from build123d import *

# Parameters (mm, degrees)
EXTRUDE086_DEPTH = 0.8
EXTRUDE087_DEPTH = 2
SKETCH084_R      = 1.8
EXTRUDE084_DEPTH = 1.6
SKETCH082_W      = 82.8
SKETCH082_H      = 36
SKETCH082_R      = 1.8
EXTRUDE082_DEPTH = 1.6
SKETCH076_R      = 7.3
EXTRUDE077_DEPTH = 1.2
SKETCH074_R      = 1.8
SKETCH074_R_2    = 6.3
EXTRUDE076_DEPTH = 2


with BuildPart() as obj1:
    # Sketch086 → Extrude086 (new body)
    with BuildSketch(Plane(origin=(0, 0, 2), x_dir=(1, 0, 0), z_dir=(0, -1, 0))):
        with BuildLine():
            Line((-137.814627, 37.2), (-142.792829, 21.878669))
            Line((-117.972457, 21.878669), (-142.792829, 21.878669))
            ThreePointArc((-117.972457, 21.878669), (-116.209101, 22.451618), (-115.119287, 23.951618))
            Line((-110.814627, 37.2), (-115.119287, 23.951618))
            Line((-137.814627, 37.2), (-110.814627, 37.2))
        make_face()
    extrude(amount=-EXTRUDE086_DEPTH)


with BuildPart() as obj1_1:
    # Extrude086 placement: moved
    add(obj1.part.moved(Location((0, 2, 0))))


with BuildPart() as extrude087:
    # Sketch087 → Extrude087 (new body)
    with BuildSketch(Plane.XZ):
        with BuildLine():
            Line((-181.329747, 20.074442), (-144.028897, 20.074442))
            Line((-137.814627, 39.2), (-144.028897, 20.074442))
            Line((-178.753577, 39.2), (-137.814627, 39.2))
            Line((-178.753577, 39.2), (-180.790744, 33.602929))
            ThreePointArc((-184.079668, 31.3), (-182.07215, 31.932968), (-180.790744, 33.602929))
            Line((-184.079668, 31.3), (-186.138695, 31.3))
            Line((-186.138695, 31.3), (-190.224464, 20.074442))
            Line((-181.329747, 20.074442), (-190.224464, 20.074442))
        make_face()
    extrude(amount=-EXTRUDE087_DEPTH)


with BuildPart() as extrude087_1:
    # Extrude087 placement: moved
    add(extrude087.part.moved(Location((0, 2, 0))))


with BuildPart() as extrude084:
    # Sketch084 → Extrude084 (new body)
    with BuildSketch(Plane.XZ):
        with BuildLine():
            ThreePointArc((-78.51, 31.3), (-76.035126, 32.325126), (-75.01, 34.8))
            Line((-75.01, 39.2), (-75.01, 34.8))
            Line((-82.8, 39.2), (-75.01, 39.2))
            Line((-82.8, 31.3), (-82.8, 39.2))
            Line((-82.8, 31.3), (-78.51, 31.3))
        make_face()
        with Locations((-78.51, 34.8)):
            Circle(SKETCH084_R, mode=Mode.SUBTRACT)
        with BuildLine():
            ThreePointArc((-9.1, 34.8), (-8.074874, 32.325126), (-5.6, 31.3))
            Line((-5.6, 31.3), (0, 31.3))
            Line((0, 39.2), (0, 31.3))
            Line((-9.1, 39.2), (0, 39.2))
            Line((-9.1, 39.2), (-9.1, 34.8))
        make_face()
        with Locations((-5.6, 34.8)):
            Circle(SKETCH084_R, mode=Mode.SUBTRACT)
        with BuildLine():
            ThreePointArc((-75.01, 7.6), (-76.035126, 10.074874), (-78.51, 11.1))
            Line((-82.8, 11.1), (-78.51, 11.1))
            Line((-82.8, 3.2), (-82.8, 11.1))
            Line((-75.01, 3.2), (-82.8, 3.2))
            Line((-75.01, 7.6), (-75.01, 3.2))
        make_face()
        with Locations((-78.51, 7.6)):
            Circle(SKETCH084_R, mode=Mode.SUBTRACT)
        with BuildLine():
            ThreePointArc((-5.6, 11.1), (-8.074874, 10.074874), (-9.1, 7.6))
            Line((-9.1, 7.6), (-9.1, 3.2))
            Line((0, 3.2), (-9.1, 3.2))
            Line((0, 11.1), (0, 3.2))
            Line((0, 11.1), (-5.6, 11.1))
        make_face()
        with Locations((-5.6, 7.6)):
            Circle(SKETCH084_R, mode=Mode.SUBTRACT)
    extrude(amount=-EXTRUDE084_DEPTH)


with BuildPart() as extrude084_1:
    # Extrude084 placement: moved
    add(extrude084.part.moved(Location((0, 2, 0))))


with BuildPart() as cut047:
    # Sketch082 → Extrude082 (new body)
    with BuildSketch(Plane.XZ):
        with Locations((-41.4, 21.2)):
            Rectangle(SKETCH082_W, SKETCH082_H)
        with Locations((-78.51, 34.8)):
            Circle(SKETCH082_R, mode=Mode.SUBTRACT)
        with Locations((-5.6, 34.8)):
            Circle(SKETCH082_R, mode=Mode.SUBTRACT)
        with Locations((-5.6, 7.6)):
            Circle(SKETCH082_R, mode=Mode.SUBTRACT)
        with Locations((-78.51, 7.6)):
            Circle(SKETCH082_R, mode=Mode.SUBTRACT)
        with BuildLine():
            ThreePointArc((-65, 31.2), (-75, 21.2), (-65, 11.2))
            Line((-65, 11.2), (-19, 11.2))
            ThreePointArc((-19, 11.2), (-9, 21.2), (-19, 31.2))
            Line((-65, 31.2), (-19, 31.2))
        make_face(mode=Mode.SUBTRACT)
    extrude(amount=-EXTRUDE082_DEPTH)


with BuildPart() as cut047_1:
    # Extrude082 placement: moved
    add(cut047.part.moved(Location((0, 2, 0))))

    # Cut047: cut Extrude084
    add(extrude084_1.part, mode=Mode.SUBTRACT)


with BuildPart() as obj2:
    # Sketch076 → Extrude077 (new body)
    with BuildSketch(Plane.XZ):
        with Locations((-65, 21.2)):
            Circle(SKETCH076_R)
        with Locations((-42, 21.2)):
            Circle(SKETCH076_R)
        with Locations((-19, 21.2)):
            Circle(SKETCH076_R)
    extrude(amount=-EXTRUDE077_DEPTH)


with BuildPart() as fusion007:
    # Sketch074 → Extrude076 (new body)
    with BuildSketch(Plane.XZ):
        with BuildLine():
            Line((-82.8, 3.2), (0, 3.2))
            Line((0, 3.2), (0, 39.2))
            Line((-195.886839, 39.2), (0, 39.2))
            Line((-202.764796, 20.302968), (-195.886839, 39.2))
            ThreePointArc((-192.175575, -3.18451), (-192.085048, 10.987093), (-202.764796, 20.302968))
            Line((-192.175575, -3.18451), (-215.419579, -53.031439))
            ThreePointArc((-215.419579, -53.031439), (-218.578907, -66.677212), (-215.93199, -80.431568))
            Line((-215.93199, -80.431568), (-176.68528, -80.431568))
            Line((-147.645309, 8.944272), (-176.68528, -80.431568))
            ThreePointArc((-132.428405, 20), (-141.832969, 16.944272), (-147.645309, 8.944272))
            Line((-132.428405, 20), (-107.6, 20))
            ThreePointArc((-91.751972, 6.2), (-97.09286, 16.066483), (-107.6, 20))
            Line((-82.8, 6.2), (-91.751972, 6.2))
            Line((-82.8, 3.2), (-82.8, 6.2))
        make_face()
        with Locations((-213.443268, -76.831568)):
            Circle(SKETCH074_R, mode=Mode.SUBTRACT)
        with Locations((-179.304663, -76.831568)):
            Circle(SKETCH074_R, mode=Mode.SUBTRACT)
        with Locations((-184.079668, 34.8)):
            Circle(SKETCH074_R, mode=Mode.SUBTRACT)
        with Locations((-78.51, 34.8)):
            Circle(SKETCH074_R, mode=Mode.SUBTRACT)
        with Locations((-78.51, 7.6)):
            Circle(SKETCH074_R, mode=Mode.SUBTRACT)
        with Locations((-5.6, 34.8)):
            Circle(SKETCH074_R, mode=Mode.SUBTRACT)
        with Locations((-5.6, 7.6)):
            Circle(SKETCH074_R, mode=Mode.SUBTRACT)
        with Locations((-19, 21.2)):
            Circle(SKETCH074_R_2, mode=Mode.SUBTRACT)
        with Locations((-42, 21.2)):
            Circle(SKETCH074_R_2, mode=Mode.SUBTRACT)
        with Locations((-65, 21.2)):
            Circle(SKETCH074_R_2, mode=Mode.SUBTRACT)
        Polygon((-189.938695, 31.567195), (-192.332836, 24.989347), (-196.467483, 26.494236), (-194.073342, 33.072084), (-193.885404, 33.00368), (-190.126633, 31.635599), align=None, mode=Mode.SUBTRACT)
    extrude(amount=-EXTRUDE076_DEPTH)

    # Cut044: cut obj2
    add(obj2.part, mode=Mode.SUBTRACT)

    # Fusion005: union Cut047
    add(cut047_1.part)

    # Fusion007: union obj1, Extrude087
    add(obj1_1.part)
    add(extrude087_1.part)


solid = fusion007.part
Here's how the part is built. I have some questions about the finished solid (model axes, mm). A direction names the side the tool comes from. Coordinates: 2 decimals unless noted, no trailing zeros. Write each loop counter-clockwise with the first axis right and the second up, starting at its lowest first coordinate (ties: lowest second). Pieces come first, ordered by that corner, then holes.
Item 1: I want a section at D-D on z = -38. Write out the boundary of the cut face in (x, y).
Item 2: If we mould it in two halves opening along Z, with no side actions, what happens to faces 1 (the flat face through (-112.937, 2.394, 32.669)), 2 (the flat face through (-188.15, 2.99, 25.77)), 3 (the cylindrical face through (-49.293, 0.592, 21.521)), 4 (the flat face through (-50, 2, 21))? For each: +Z half, -Z half, draft (parallel to the pull), parting line (faces both ways), or undercut.
Item 3: I want a section at B-B on x = -170.5. Write out the boundary of the cut face in (y, z).
Item 4: I want a section at C-C on z = -68. Write out the boundary of the cut face in (x, y).
Item 5: If I drill on line 1 (Z direction, x = -5.6, y = 1.35); line 2 (Z direction, x = -65, y = 0.55); line 3 (Z direction, x = -42, y = 1.75), over which ranges is the centre line in solid material (lowest first)?
Item 6: On a 3-axis mill with a long thin cutter (end or side, diameter ignored), from which of +Z, -Z, +X, -X, +Y, -Y can I reach the whole of each face in a straight line? I mean faces 5 (the cylindrical face through (-141.719, 0.986, 17.026)), 6 (the flat face through (-39, 1.2, 27)), 7 (the flat face through (-141.569, 3.208, 27.646)), 8 (the flat face through (-3.6, 2, 7.2)). Say none if no direction works.
Item 7: Will these pins go through, and if not, where does the flat tip stop? pin 1 (0.8 mm diameter, centred on x = -80, y = 3, fed in from +Z); pin 2 (0.5 mm diameter, centred on y = 3, z = 6, fed in from +X); pin 3 (4 mm diameter, centred on x = -4.5, z = 34, fed in from +Y); pin 4 (3 mm diameter, centred on x = -5.6, z = 34.8, fed in from -Y).
Item 8: I want a section at A-A on x = -42. Write out the boundary of the cut face in (y, z).
Findings below:
1. outline: (-208.41, 0) - (-162.9, 0) - (-162.9, 2) - (-208.41, 2) - close
2. face 1: -Z half
2. face 2: +Z half
2. face 3: undercut
2. face 4: undercut
3. outline: (0, -61.4) - (2, -61.4) - (2, 20.07) - (4, 20.07) - (4, 39.2) - (0, 39.2) - close
4. outline: (-218.58, 0) - (-172.65, 0) - (-172.65, 2) - (-218.58, 2) - close
5. line 1: z = 3.2 to 5.8, 9.4 to 33, 36.6 to 39.2
5. line 2: z = 3.2 to 13.9, 28.5 to 39.2
5. line 3: z = 3.2 to 14.9, 27.5 to 39.2
6. face 5: -Z, +Y, -Y
6. face 6: -Y
6. face 7: -Z, +Y
6. face 8: -Z, +X, +Y
7. pin 1: stops at z = 31.3
7. pin 2: stops at x = -9.1
7. pin 3: stops at y = 2
7. pin 4: passes through
8. outline: (0, 3.2) - (3.6, 3.2) - (3.6, 11.2) - (2, 11.2) - (2, 14.9) - (1.2, 14.9) - (1.2, 13.9) - (0, 13.9) - close; (0, 28.5) - (1.2, 28.5) - (1.2, 27.5) - (2, 27.5) - (2, 31.2) - (3.6, 31.2) - (3.6, 39.2) - (0, 39.2) - close
